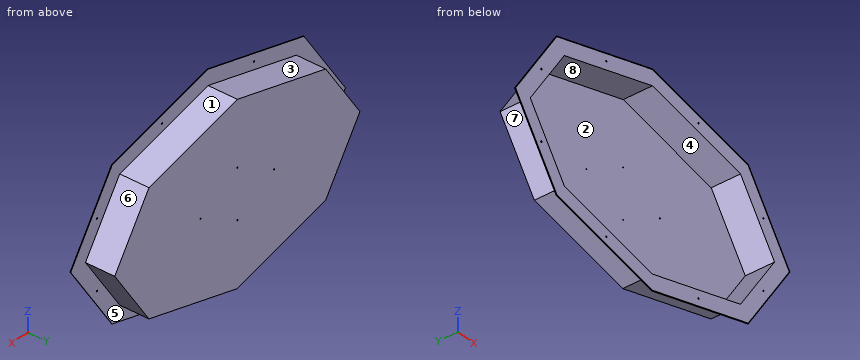
from build123d import *

# Parameters (mm, degrees)
BOSS_EXTRUDE1_DEPTH   = 152.4
BOSS_EXTRUDE2_DEPTH   = 3.175
SHELL1_T              = -2.38125
SKETCH3_R             = 3.175
CUT_EXTRUDE1_DEPTH    = 1020.94798284
CRVPATTERN1_START     = 150.01875
CRVPATTERN1_OUTLINE_R = 3.175
CRVPATTERN1_DEPTH     = 2.38125
CUT_EXTRUDE2_REACH    = 1021.469
SKETCH5_R             = 3.81


# Read off the part's stored shape, not the designer's step: CrvPattern1
with BuildPart() as part:
    # Sketch1 → Boss-Extrude1 (new body)
    with BuildSketch(Plane(origin=(0, 0, 0), x_dir=(1, 0, 0), z_dir=(0, 1, 0))):
        Polygon((-549.079439398, 317.011162143), (0, 457.2), (549.079439398, 317.011162143), (762, 0), (549.079439398, -317.011162143), (0, -457.2), (-549.079439398, -317.011162143), (-762, 0), align=None)
    extrude(amount=BOSS_EXTRUDE1_DEPTH)

    # Sketch2 → Boss-Extrude2 (add)
    with BuildSketch(Plane.XZ):
        Polygon((0, 535.844392641), (-596.116107134, 383.646334781), (-853.792184287, 0), (-596.116107134, -383.646334781), (0, -535.844392641), (596.116107134, -383.646334781), (853.792184287, 0), (596.116107134, 383.646334781), align=None)
    extrude(amount=BOSS_EXTRUDE2_DEPTH)

    # Shell1
    shell1_openings = [part.faces().sort_by_distance(p)[0] for p in [
        (0, -3.175, 0),
    ]]
    offset(amount=SHELL1_T, openings=shell1_openings, kind=Kind.INTERSECTION)

    # Sketch3 → Cut-Extrude1 (cut, through all)
    with BuildSketch(Plane(origin=(0, 152.4, 0), x_dir=(1, 0, 0), z_dir=(0, 1, 0))):
        with Locations(Location((0, 127, 0), (0, 0, 270))):
            Circle(SKETCH3_R)
    extrude(amount=-CUT_EXTRUDE1_DEPTH, mode=Mode.SUBTRACT)

    # CrvPattern1 outline → CrvPattern1 (cut)
    with BuildSketch(Plane(origin=(0, 0, 0), x_dir=(1, 0, 0), z_dir=(0, 1, 0)).offset(CRVPATTERN1_START)):
        with Locations((-228.6, 0)):
            Circle(CRVPATTERN1_OUTLINE_R)
        with Locations((0, -127)):
            Circle(CRVPATTERN1_OUTLINE_R)
        with Locations((228.6, 0)):
            Circle(CRVPATTERN1_OUTLINE_R)
    extrude(amount=CRVPATTERN1_DEPTH, mode=Mode.SUBTRACT)

    # Sketch5 → Cut-Extrude2 (cut, up to next)
    with BuildSketch(Plane(origin=(0, 0, 0), x_dir=(1, 0, 0), z_dir=(0, 1, 0)), mode=Mode.PRIVATE) as cut_extrude2_sk1:
        with Locations(Location((-286.298886633, 423.425472391, 0), (0, 0, 270))):
            Circle(SKETCH5_R)
    cut_extrude2_tool1 = extrude(cut_extrude2_sk1.sketch, amount=-CUT_EXTRUDE2_REACH, mode=Mode.PRIVATE) & part.part
    # Sketch5 → Cut-Extrude2 (cut, up to next)
    with BuildSketch(Plane(origin=(0, 0, 0), x_dir=(1, 0, 0), z_dir=(0, 1, 0)), mode=Mode.PRIVATE) as cut_extrude2_sk2:
        with Locations(Location((-690.246932705, 175.164374231, 0), (0, 0, 270))):
            Circle(SKETCH5_R)
    cut_extrude2_tool2 = extrude(cut_extrude2_sk2.sketch, amount=-CUT_EXTRUDE2_REACH, mode=Mode.PRIVATE) & part.part
    # Sketch5 → Cut-Extrude2 (cut, up to next)
    with BuildSketch(Plane(origin=(0, 0, 0), x_dir=(1, 0, 0), z_dir=(0, 1, 0)), mode=Mode.PRIVATE) as cut_extrude2_sk3:
        with Locations(Location((-690.246932705, -175.164374231, 0), (0, 0, 270))):
            Circle(SKETCH5_R)
    cut_extrude2_tool3 = extrude(cut_extrude2_sk3.sketch, amount=-CUT_EXTRUDE2_REACH, mode=Mode.PRIVATE) & part.part
    # Sketch5 → Cut-Extrude2 (cut, up to next)
    with BuildSketch(Plane(origin=(0, 0, 0), x_dir=(1, 0, 0), z_dir=(0, 1, 0)), mode=Mode.PRIVATE) as cut_extrude2_sk4:
        with Locations(Location((-286.298886633, -423.425472391, 0), (0, 0, 270))):
            Circle(SKETCH5_R)
    cut_extrude2_tool4 = extrude(cut_extrude2_sk4.sketch, amount=-CUT_EXTRUDE2_REACH, mode=Mode.PRIVATE) & part.part
    # Sketch5 → Cut-Extrude2 (cut, up to next)
    with BuildSketch(Plane(origin=(0, 0, 0), x_dir=(1, 0, 0), z_dir=(0, 1, 0)), mode=Mode.PRIVATE) as cut_extrude2_sk5:
        with Locations(Location((286.298886633, -423.425472391, 0), (0, 0, 270))):
            Circle(SKETCH5_R)
    cut_extrude2_tool5 = extrude(cut_extrude2_sk5.sketch, amount=-CUT_EXTRUDE2_REACH, mode=Mode.PRIVATE) & part.part
    # Sketch5 → Cut-Extrude2 (cut, up to next)
    with BuildSketch(Plane(origin=(0, 0, 0), x_dir=(1, 0, 0), z_dir=(0, 1, 0)), mode=Mode.PRIVATE) as cut_extrude2_sk6:
        with Locations(Location((690.246932705, -175.164374231, 0), (0, 0, 270))):
            Circle(SKETCH5_R)
    cut_extrude2_tool6 = extrude(cut_extrude2_sk6.sketch, amount=-CUT_EXTRUDE2_REACH, mode=Mode.PRIVATE) & part.part
    # Sketch5 → Cut-Extrude2 (cut, up to next)
    with BuildSketch(Plane(origin=(0, 0, 0), x_dir=(1, 0, 0), z_dir=(0, 1, 0)), mode=Mode.PRIVATE) as cut_extrude2_sk7:
        with Locations(Location((690.246932705, 175.164374231, 0), (0, 0, 270))):
            Circle(SKETCH5_R)
    cut_extrude2_tool7 = extrude(cut_extrude2_sk7.sketch, amount=-CUT_EXTRUDE2_REACH, mode=Mode.PRIVATE) & part.part
    # Sketch5 → Cut-Extrude2 (cut, up to next)
    with BuildSketch(Plane(origin=(0, 0, 0), x_dir=(1, 0, 0), z_dir=(0, 1, 0)), mode=Mode.PRIVATE) as cut_extrude2_sk8:
        with Locations(Location((286.298886633, 423.425472391, 0), (0, 0, 270))):
            Circle(SKETCH5_R)
    cut_extrude2_tool8 = extrude(cut_extrude2_sk8.sketch, amount=-CUT_EXTRUDE2_REACH, mode=Mode.PRIVATE) & part.part
    add(cut_extrude2_tool1.solids().sort_by_distance((-286.298887, 0, -423.425472))[0], mode=Mode.SUBTRACT)
    add(cut_extrude2_tool2.solids().sort_by_distance((-690.246933, 0, -175.164374))[0], mode=Mode.SUBTRACT)
    add(cut_extrude2_tool3.solids().sort_by_distance((-690.246933, 0, 175.164374))[0], mode=Mode.SUBTRACT)
    add(cut_extrude2_tool4.solids().sort_by_distance((-286.298887, 0, 423.425472))[0], mode=Mode.SUBTRACT)
    add(cut_extrude2_tool5.solids().sort_by_distance((286.298887, 0, 423.425472))[0], mode=Mode.SUBTRACT)
    add(cut_extrude2_tool6.solids().sort_by_distance((690.246933, 0, 175.164374))[0], mode=Mode.SUBTRACT)
    add(cut_extrude2_tool7.solids().sort_by_distance((690.246933, 0, -175.164374))[0], mode=Mode.SUBTRACT)
    add(cut_extrude2_tool8.solids().sort_by_distance((286.298887, 0, -423.425472))[0], mode=Mode.SUBTRACT)


solid = part.part
Source: CAD feature listing. Evaluate the final solid. Frame: model axes, mm. Face numbers are marked on the shaded views. A direction names the side the tool comes from. Give positions to 0.01 mm unless a question says otherwise; leave off trailing zeros. Write each loop counter-clockwise with the first axis right and the second up, starting at its lowest first coordinate (ties: lowest second). Pieces come first, ordered by that corner, then holes. Notation, with made-up numbers: M 68,51.5 L 72,51.5 A12 ccw 72,72.5 Z; hole C 28,33 d9. An arc over 180 degrees is marked long. Return JSON: item names as keys, results as strings. Group by question number.
1) Draft query along X for the marked faces 1, 2, 3 and 4. Return one class per face: released by +X, released by -X, zero draft, split by the parting line, or undercut.
2) Set-up query: the marked faces 5, 6, 7 and 8. Return all of +Z, -Z, +X, -X, +Y, -Y with unobstructed straight access to the full face (end or side cutting, diameter ignored); none if empty.
3) First-contact query: pin 1 Ø2 at (y, z) = (108.5, -284) entering from +X; pin 2 Ø5 at (x, y) = (358.5, 89.5) entering from -Z; pin 3 Ø3 at (x, y) = (-251, 106.5) entering from +Z; pin 4 Ø7 at (x, z) = (-286.3, 423.43) entering from +Y. Flat tips, straight axial feed; report the tip coordinate or a pass-through.
4) Cut plane B-B, the plane z = -92. Output: boundary loops of the cut face in (x, y) (3 decimals), then the cut area to 3 significant figures.
5) Cut plane A-A, the plane y = 41. Output: boundary loops of the cut face in (x, z), then the cut area to 3 significant figures.
6) Cut plane C-C, the plane x = -647. Output: boundary loops of the cut face in (y, z) (3 decimals).
7) Ray query, L1, parallel to Y at x = -265.5, z = -40; L2, parallel to Z at x = 138, y = 115; L3, parallel to Z at x = 244.5, y = 36. Return the intervals inside material, ascending.
Data:
{
 "1": {"face 1": "released by +X", "face 2": "undercut", "face 3": "released by -X", "face 4": "undercut"},
 "2": {"face 5": "+Y", "face 6": "+Z, +X, +Y", "face 7": "-Z, -X, +Y", "face 8": "-Y"},
 "3": {"pin 1": "stops at x = 571.92", "pin 2": "stops at z = -366.31", "pin 3": "stops at z = 393.5", "pin 4": "passes through"},
 "4": {"outline": "M -792,-3.175 L -789.132,-3.175 L -789.132,-2.381 L -697.34,-2.381 L -697.34,150.019 L 697.34,150.019 L 697.34,-2.381 L 789.132,-2.381 L 789.132,-3.175 L 792,-3.175 L 792,0 L 700.208,0 L 700.208,152.4 L -700.208,152.4 L -700.208,0 L -792,0 Z", "area": "4,650 mm²"},
 "5": {"outline": "M -762,0 L -549.08,-317.01 L 0,-457.2 L 549.08,-317.01 L 762,0 L 549.08,317.01 L 0,457.2 L -549.08,317.01 Z; hole M -759.13,0 L -547.61,-314.93 L 0,-454.74 L 547.61,-314.93 L 759.13,0 L 547.61,314.93 L 0,454.74 L -547.61,314.93 Z", "area": "9,020 mm²"},
 "6": {"outline": "M -3.175,-307.887 L 0,-307.887 L 0,-171.22 L 152.4,-171.22 L 152.4,171.22 L 0,171.22 L 0,307.887 L -3.175,307.887 L -3.175,303.616 L -2.381,303.616 L -2.381,166.949 L 150.019,166.949 L 150.019,-166.949 L -2.381,-166.949 L -2.381,-303.616 L -3.175,-303.616 Z"},
 "7": {"L1": "y = 150.02 to 152.4", "L2": "z = -421.97 to -419.51, 419.51 to 421.97", "L3": "z = -394.78 to -392.32, 392.32 to 394.78"}
}
